Part model, mm, in its own coordinate system. A direction names the side the tool comes from. Give positions to 0.01 mm unless a question says otherwise; leave off trailing zeros. Order: outer loops, then holes, each group sorted by start corner. A loop starts at its lowest first (then second) coordinate and runs counter-clockwise, first axis right, second up. Notation, with made-up numbers: M -3,36.25 L 1,36.25 A30 ccw 1,65.25 Z; hole C -16,53 d4. An arc over 180 degrees is marked long. Return JSON: item names as keys, results as strings.
from build123d import *

# Parameters (mm, degrees)
SKETCH50_R         = 1.75
EXTRUDE1_DEPTH     = 8
SKETCH52_R         = 4.15
SKETCH52_R_2       = 1.7
EXTRUDE2_DEPTH     = 7
FILLET1_R          = 3
FILLET2_R          = 5
EXTRUDE3_DEPTH     = 4.5
FILLET4_R          = 5
FILLET5_R          = 3
SKETCH55_R         = 3
CUT_EXTRUDE3_DEPTH = 4
FILLET9_R          = 1
FILLET10_R         = 1
SKETCH57_W         = 1
SKETCH57_H         = 8.155835086
EXTRUDE4_DEPTH     = 4
CUT_EXTRUDE4_START = -7
SKETCH56_W         = 0.996940693
SKETCH56_H         = 2.63977817
CUT_EXTRUDE4_DEPTH = 7.000001


with BuildPart() as part:
    # Sketch50 → Extrude1 (new body)
    with BuildSketch(Plane(origin=(60, 0, 0), x_dir=(0, 0, -1), z_dir=(1, 0, 0))):
        Polygon((-38.234887292, -28), (-38.234887292, -38), (-15, -55.32486375), (0, -55.32486375), (0, -8.32486375), (-15, -8.32486375), align=None)
        with Locations((-35, -33)):
            Circle(SKETCH50_R, mode=Mode.SUBTRACT)
        with Locations((-15, -23)):
            Circle(SKETCH50_R, mode=Mode.SUBTRACT)
        with Locations((-15, -43)):
            Circle(SKETCH50_R, mode=Mode.SUBTRACT)
    extrude(amount=EXTRUDE1_DEPTH)

    # Sketch52 → Extrude2 (add)
    with BuildSketch(Plane(origin=(0, 0, 0), x_dir=(-1, 0, 0), z_dir=(0, 0, -1))):
        Polygon((-61.521067729, -55.328445544), (-61.521067729, -8.328445544), (-112.5, -8.328445544), (-112.5, -22.280627193), (-77.5, -22.280627193), (-77.5, -55.328445544), align=None)
        with Locations(Location((-89.299980942, -17.200015896, 0), (0, 0, 90))):
            Circle(SKETCH52_R, mode=Mode.SUBTRACT)
        with Locations(Location((-73.351535893, -18.931266408, 0), (0, 0, 90))):
            Circle(SKETCH52_R_2, mode=Mode.SUBTRACT)
        with Locations(Location((-104.8, -18.5, 0), (0, 0, 90))):
            Circle(SKETCH52_R_2, mode=Mode.SUBTRACT)
        with Locations(Location((-73.801481725, -49.508569042, 0), (0, 0, 90))):
            Circle(SKETCH52_R_2, mode=Mode.SUBTRACT)
    extrude(amount=-EXTRUDE2_DEPTH)

    # Fillet1
    fillet1_edges = [part.edges().sort_by_distance(p)[0] for p in [
        (112.5, -22.280627193, 3.5),
        (112.5, -8.328445544, 3.5),
    ]]
    fillet(fillet1_edges, radius=FILLET1_R)

    # Fillet2
    fillet2_edges = [part.edges().sort_by_distance(p)[0] for p in [
        (77.5, -55.328445544, 3.5),
    ]]
    fillet(fillet2_edges, radius=FILLET2_R)

    # Sketch54 → Extrude3 (add)
    with BuildSketch(Plane(origin=(0, -8.328445544, 0), x_dir=(1, 0, 0), z_dir=(0, 1, 0))):
        with BuildLine():
            Line((68, -15), (68, -7))
            Line((68, -7), (84.179453899, -7))
            ThreePointArc((84.179453899, -7), (75.154838555, -9.109252039), (68, -15))
        make_face()
    extrude(amount=-EXTRUDE3_DEPTH)

    # Fillet4
    fillet4_edges = [part.edges().sort_by_distance(p)[0] for p in [
        (64, -55.32486375, 15),
        (64, -38, 38.234887292),
        (64, -28, 38.234887292),
    ]]
    fillet(fillet4_edges, radius=FILLET4_R)

    # Fillet5
    fillet5_edges = [part.edges().sort_by_distance(p)[0] for p in [
        (60, -8.32486375, 7.5),
    ]]
    fillet(fillet5_edges, radius=FILLET5_R)

    # Sketch55 → Cut-Extrude3 (cut)
    with BuildSketch(Plane(origin=(68, 0, 0), x_dir=(0, 0, -1), z_dir=(1, 0, 0))):
        with Locations((-15, -23)):
            Circle(SKETCH55_R)
        with Locations((-15, -43)):
            Circle(SKETCH55_R)
        with BuildLine():
            Line((-35, -30), (-38.787900912, -30))
            Line((-38.787900912, -30), (-38.787900912, -36))
            Line((-38.787900912, -36), (-35, -36))
            ThreePointArc((-35, -36), (-32, -33), (-35, -30))
        make_face()
    extrude(amount=-CUT_EXTRUDE3_DEPTH, mode=Mode.SUBTRACT)

    # Fillet9
    # the kernel refuses this fillet: 1 mm, written as the material it takes off along each edge
    with BuildSketch(Plane(origin=(89.299980942, -17.200015896, 0), x_dir=(0, 1, 0), z_dir=(-1, 0, 0))) as fillet9_piece_1:
        with BuildLine():
            CenterArc((4.15 + FILLET9_R, -FILLET9_R), FILLET9_R, 90, 90)
            Line((4.15, -FILLET9_R), (4.15, 0))
            Line((4.15, 0), (4.15 + FILLET9_R, 0))
        make_face()
    revolve(axis=Axis((89.299980942, -17.200015896, 0), (0, 0, -1)), mode=Mode.SUBTRACT)

    # Fillet10
    # the kernel refuses this fillet: 1 mm, written as the material it takes off along each edge
    with BuildSketch(Plane(origin=(89.299980942, -17.200015896, 7), x_dir=(0, 1, 0), z_dir=(-1, 0, 0))) as fillet10_piece_1:
        with BuildLine():
            CenterArc((4.15 + FILLET10_R, FILLET10_R), FILLET10_R, 180, 90)
            Line((4.15, FILLET10_R), (4.15, 0))
            Line((4.15, 0), (4.15 + FILLET10_R, 0))
        make_face()
    revolve(axis=Axis((89.299980942, -17.200015896, 7), (0, 0, -1)), mode=Mode.SUBTRACT)

    # Sketch57 → Extrude4 (cut)
    with BuildSketch(Plane.XZ.offset(22.280627193)):
        with Locations((89.327585964, 3.449545077)):
            Rectangle(SKETCH57_W, SKETCH57_H)
    extrude(amount=-EXTRUDE4_DEPTH, mode=Mode.SUBTRACT)

    # Sketch56 → Cut-Extrude4 (cut)
    with BuildSketch(Plane(origin=(0, 0, 0), x_dir=(-1, 0, 0), z_dir=(0, 0, -1)).offset(CUT_EXTRUDE4_START)):
        with Locations((-88.818861809, -22.280627193)):
            Rectangle(SKETCH56_W, SKETCH56_H)
    extrude(amount=CUT_EXTRUDE4_DEPTH, mode=Mode.SUBTRACT)


solid = part.part
Q1. Probe line 1 along Y through (x, z) = (65.7, 15); line 2 along X through (y, z) = (-29.5, 31.5); line 3 along X through (y, z) = (-18, 3). List the from-to ranges inside material, lowest first.
Established:
{"line 1": "y = -55.04 to -46, -40 to -26, -20 to -8.32", "line 2": "x = 60 to 68", "line 3": "x = 60 to 71.93, 74.77 to 85.23, 93.37 to 103.18, 106.42 to 112.5"}
Q2. 3-axis set-ups, long thin cutter, end or side, ignore diameter. For faces 4 (the cylindrical face through (61.97, -31.82, 36.29)), 5 (the flat face through (100, -22.281, 3)), 6 (the cylindrical face through (66, -33, 32)), 7 (the flat face through (64, -45, 15)): which of +Z, -Z, +X, -X, +Y, -Y reach the whole face in a straight line?
Established:
{"face 4": "+X, -X", "face 5": "+Z, -Z, +X, -Y", "face 6": "+Z, +X", "face 7": "+X"}
Q3. Band-saw the part on A-A (z = 34). Give the cut face in (x, y), then the cut area to 3 significant figures.
Established:
{"outline": "M 60,-41.16 L 68,-41.16 L 68,-35.83 L 64,-35.83 L 64,-34.44 L 60,-34.44 Z; M 60,-31.56 L 64,-31.56 L 64,-30.17 L 68,-30.17 L 68,-24.41 L 60,-24.41 Z", "area": "99.8 mm²"}
Q4. Pin check, flat tips, straight feed: pin 1 (3.5 mm diameter, centred on x = 96, z = 3, fed in from -Y); pin 2 (5.5 mm diameter, centred on y = -23, z = 15, fed in from -X); pin 3 (4.5 mm diameter, centred on x = 104.8, y = -18.5, fed in from +Z); pin 4 (9 mm diameter, centred on x = 78.5, z = 9, fed in from -Y). Stop position of each tip, or through.
Established:
{"pin 1": "stops at y = -22.28", "pin 2": "stops at x = 60", "pin 3": "stops at z = 7", "pin 4": "stops at y = -54.92"}
Q5. Band-saw the part on B-B (y = -43). Give the cut face in (x, z).
Established:
{"outline": "M 60,0 L 77.5,0 L 77.5,7 L 68,7 L 68,12 L 64,12 L 64,13.25 L 60,13.25 Z; M 60,16.75 L 64,16.75 L 64,18 L 68,18 L 68,31.53 L 60,31.53 Z"}
Q6. Band-saw the part on C-C (y = -23). Give the cut face in (x, z), then the cut area to 3 significant figures.
Established:
{"outline": "M 60,0 L 77.5,0 L 77.5,7 L 68,7 L 68,12 L 64,12 L 64,13.25 L 60,13.25 Z; M 60,16.75 L 64,16.75 L 64,18 L 68,18 L 68,32.33 L 60,32.33 Z", "area": "287 mm²"}
Q7. Two-plate mould, pull along Z, no slides. Class faces 1 (the cylindrical face through (61.97, -44.71, 15.38)), 2 (the flat face through (63, -55.325, 10)), 3 (the cylindrical face through (75.272, -10.547, 9.052)): +Z half, -Z half, draft (parallel to the pull), parting line (faces both ways), or undercut.
Established:
{"face 1": "undercut", "face 2": "draft", "face 3": "+Z half"}
